```python
from build123d import *

# Parameters (mm, degrees)
SKETCH1_R           = 2.25
BOSS_EXTRUDE1_DEPTH = 2


with BuildPart() as part:
    # Sketch1 → Boss-Extrude1 (new, symmetric)
    with BuildSketch(Plane.XY):
        with BuildLine():
            Line((0, 3.25), (20, 3.25))
            ThreePointArc((20, 3.25), (23.25, 0), (20, -3.25))
            Line((20, -3.25), (0, -3.25))
            ThreePointArc((0, -3.25), (-3.25, 0), (0, 3.25))
        make_face()
        Circle(SKETCH1_R, mode=Mode.SUBTRACT)
        with Locations((20, 0)):
            Circle(SKETCH1_R, mode=Mode.SUBTRACT)
    extrude(amount=BOSS_EXTRUDE1_DEPTH, both=True)


solid = part.part
```
The listing builds one solid part. Answer for the finished solid, in the listing's coordinates (mm). Coordinates: 2 decimals unless noted, no trailing zeros. Loops run counter-clockwise (first coordinate to the right, second up) from the corner with the lowest first, then second, coordinate; pieces in that order, holes last. Notation, with made-up numbers: M 37,42.5 L 77,42.5 A15 ccw 77,68.5 Z; hole C 73,59.5 d5. An arc over 180 degrees is marked long. Answer as a JSON object with one key per item and string values. Group by question number.
Item 1: Section C-C (y = -1.25) is taken. Write down the section's boundary in (x, z), and give its area (3 significant figures).
Item 2: Consider L1, parallel to Y at x = 0, z = -0.5; L2, parallel to X at y = 1.75, z = 1.4; L3, parallel to X at y = -1, z = 1.85. Determine where each line is inside the solid, lowest interval first.
Item 3: Determine the mould class of faces 1 (the face through (22.146, 0.676, -0.028)), 2 (the face through (23.25, 0.07, 0.03)), 3 (the face through (-3.25, -0.07, 0.03)), 4 (the face through (10, 0, 2)) for opening direction X: +X half, -X half, draft (parallel to the pull), parting line (faces both ways), or undercut.
Item 4: Section B-B (z = -1.65) is taken. Write down the section's boundary in (x, y).
Item 5: Section A-A (y = 0) is taken. Write down the section's boundary in (x, z), and give its area (3 significant figures).
Solved:
{
 "1": {"outline": "M -3,-2 L -1.87,-2 L -1.87,2 L -3,2 Z; M 1.87,-2 L 18.13,-2 L 18.13,2 L 1.87,2 Z; M 21.87,-2 L 23,-2 L 23,2 L 21.87,2 Z", "area": "74.1 mm2"},
 "2": {"L1": "y = -3.25 to -2.25, 2.25 to 3.25", "L2": "x = -2.74 to -1.41, 1.41 to 18.59, 21.41 to 22.74", "L3": "x = -3.09 to -2.02, 2.02 to 17.98, 22.02 to 23.09"},
 "3": {"face 1": "undercut", "face 2": "+X half", "face 3": "-X half", "face 4": "draft"},
 "4": {"outline": "M 0,-3.25 L 20,-3.25 A3.25 ccw 20,3.25 L 0,3.25 A3.25 ccw Z; hole C 0,0 d4.5; hole C 20,0 d4.5"},
 "5": {"outline": "M -3.25,-2 L -2.25,-2 L -2.25,2 L -3.25,2 Z; M 2.25,-2 L 17.75,-2 L 17.75,2 L 2.25,2 Z; M 22.25,-2 L 23.25,-2 L 23.25,2 L 22.25,2 Z", "area": "70.0 mm2"}
}
